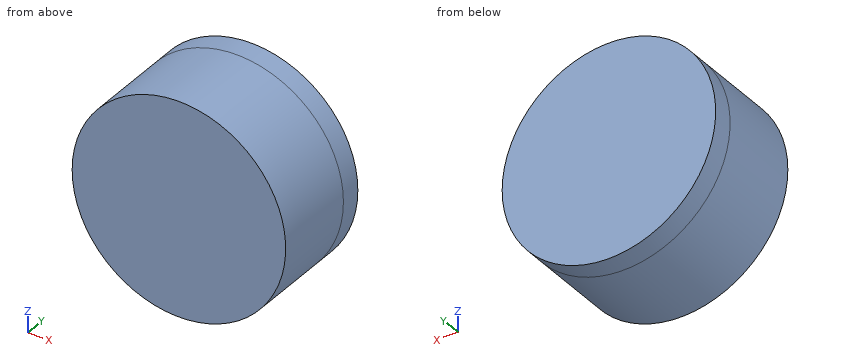
Autodesk Inventor part; units mm, degrees
ref_plane "YZ Plane" through (0, 0, 0) normal (1, 0, 0) x (0, 1, 0)
ref_plane "XZ Plane" through (0, 0, 0) normal (0, 1, 0) x (-1, 0, 0)
ref_plane "XY Plane" through (0, 0, 0) normal (0, 0, 1) x (1, 0, 0)
sketch "Sketch1" plane through (0, 0, 0) normal (0, 1, 0) x (-1, 0, 0)
  point P0 (0, 0)
sketch "Sketch2" plane through (0, 0, 0) normal (0, 1, 0) x (-1, 0, 0)
  circle A0 centre (0, 0) radius 50
  dimension "d0" = 100
extrude "Extrusion1" add sketch "Sketch2" along normal blind 10
sketch "Sketch3" plane through (0, 10, 0) normal (0, 1, 0) x (1, 0, 0)
  circle A0 centre (0, 0) radius 50
  circle A1 centre (0, 0) radius 45
  circle A2 centre (0, 0) radius 10
  dimension "d3" = 90
  dimension "d4" = 20
extrude "Extrusion2" add sketch "Sketch3" along normal blind 30
sketch "Sketch4" plane through (0, 40, 0) normal (0, 1, 0) x (1, 0, 0)
  circle A0 centre (0, 0) radius 50
extrude "Extrusion3" add sketch "Sketch4" along normal blind 10
properties part number "cyl2_10cm_5cm"
The model under review builds one solid part; all positions refer to its coordinate system, in mm. Round coordinates to 2 decimals unless told otherwise and drop trailing zeros. Loops run counter-clockwise (first coordinate to the right, second up) from the corner with the lowest first, then second, coordinate; pieces in that order, holes last. Notation, with made-up numbers: M -38,50.25 L 12,50.25 A32 ccw 12,76.25 Z; hole C 86.25,-31.75 d8. An arc over 180 degrees is marked long. Answer as CSV lines item,"result". Start each with the question number.
Item 1: Wall thickness on line 1 (Z direction, x = 0, y = 26.5); line 2 (Y direction, x = 25, z = -1.5): over which ranges is each line inside the solid? List them lowest first. Write a range as [from, to].
Item 2: Insertion check: P1, Ø1.5, axis at y = 37.5, z = 17, coming from the -X side; P2, Ø8, axis at x = -5, y = 29.5, coming from the -Z side; P3, Ø1.5, axis at x = 34, y = 43, coming from the -Z side. Each pin has a flat end and moves straight along its axis. Give the tip position at first contact, or say it passes through.
Item 3: Consider section B-B (z = -25.5). Write out the cut boundary in (x, y), then the cut area to 3 significant figures.
Item 4: Consider section A-A (y = 26). Write out the cut boundary in (x, z).
Answer:
1,line 1,"z = [-50, -45], [-10, 10], [45, 50]"
1,line 2,"y = [0, 10], [40, 50]"
2,P1,"stops at x = -47.29"
2,P2,"stops at z = -49.99"
2,P3,"stops at z = -37.34"
3,outline,"M -43.01,0 L 43.01,0 L 43.01,50 L -43.01,50 Z; hole M -37.08,10 L 37.08,10 L 37.08,40 L -37.08,40 Z"
3,area,"2,080 mm^2"
4,outline,"C 0,0 d100; C 0,0 d20; hole C 0,0 d90"
